For this review, take the finished solid that the model builds, in its own axes (mm). A direction names the side the tool comes from. Give positions to 0.01 mm unless a question says otherwise; leave off trailing zeros. Write each loop counter-clockwise with the first axis right and the second up, starting at its lowest first coordinate (ties: lowest second). Pieces come first, ordered by that corner, then holes.
Q1. For line 1 (Z direction, x = 10, y = -5.75); line 2 (Y direction, x = 14.5, z = 4.25); line 3 (X direction, y = 1, z = 14.5), list the stretches that pass through material, from the lowest coordinate up.
Q2. We need section B-B (x = 10). Write out the cut boundary in (y, z).
Q3. We need section C-C (x = -7.5). Write out the cut boundary in (y, z), then the cut area to 3 significant figures.
Q4. Mouldability with a two-part tool opening along Z and no side actions: class faces 3 (the cylindrical face through (12.75, 8.4, 9.86)), 4 (the flat face through (0, 0, 0)), 5 (the cylindrical face through (-2.899, -13.521, 10.083)), 6 (the cylindrical face through (-15.045, -13.521, 3.873)) as released by +Z, released by -Z, zero draft, split by the parting line, or undercut.
Q5. We need section A-A (z = 10.5). Give the number of separate pieces and of enclosed holes in the cut face, then the cut area to 3 significant figures.
Q6. Machinability: for faces 1 (the cylindrical face through (12.85, -8.04, 9.86)), 2 (the flat face through (0, 2, 11)), which of the approach directions +Z, -Z, +X, -X, +Y, -Y give a long, thin tool a straight path to every point of the face, cutting with its end or side? Answer none if there is none.
Q7. Insertion check: P1, Ø5.5, axis at x = -14.4, z = 6.8, coming from the +Y side; P2, Ø16, axis at x = -14.5, y = 3.5, coming from the +Z side; P3, Ø1, axis at y = -10, z = 11, coming from the -X side. Each pin has a flat end and moves straight along its axis. Give the tip position at first contact, or say it passes through.
Q8. We need section D-D (x = 6). Write out the cut boundary in (y, z).
```python
from build123d import *

# Parameters (mm, degrees)
F0_W     = 20
F0_H     = 27
F0_R     = 3
F0_R_2   = 2.75
F0_R_3   = 2.5
F1_DEPTH = 3
F0_R_4   = 1.55
F0_R_5   = 1.6
F0_R_6   = 1.5
F0_R_7   = 1.65
F0_R_8   = 1.45
F0_R_9   = 1.7
F2_DEPTH = 20
F0_H_2   = 3
F3_DEPTH = 20
F4_R     = 1.4
F4_R_2   = 1.45
F4_R_3   = 1.5
F4_R_4   = 2.75
F4_R_5   = 2.5
F4_R_6   = 3
F5_DEPTH = 30


with BuildPart() as f1:
    # F0 (on Top) → F1 (new body)
    with BuildSketch(Plane.XY):
        with Locations((-10, 1.5)):
            Rectangle(F0_W, F0_H)
        with Locations((-13.873821, -1.985078)):
            Circle(F0_R, mode=Mode.SUBTRACT)
        with Locations((-5.548216, 2.859571)):
            Circle(F0_R_2, mode=Mode.SUBTRACT)
        with Locations((-13.873821, 8.230659)):
            Circle(F0_R_3, mode=Mode.SUBTRACT)
    extrude(amount=F1_DEPTH)

    # F0 (on Top) → F2 (join)
    with BuildSketch(Plane.XY):
        Polygon((0, -15), (20, -15), (20, 15), (0, 15), (0, -12), align=None)
        with Locations((6.521292, -8.111834)):
            Circle(F0_R_4, mode=Mode.SUBTRACT)
        with Locations((14.447207, -8.111834)):
            Circle(F0_R_5, mode=Mode.SUBTRACT)
        with Locations((6.521292, 0)):
            Circle(F0_R_6, mode=Mode.SUBTRACT)
        with Locations((14.447207, 0)):
            Circle(F0_R_7, mode=Mode.SUBTRACT)
        with Locations((6.521292, 8.330117)):
            Circle(F0_R_8, mode=Mode.SUBTRACT)
        with Locations((14.447207, 8.330117)):
            Circle(F0_R_9, mode=Mode.SUBTRACT)
    extrude(amount=F2_DEPTH)

    # F0 (on Top) → F3 (join, through all)
    with BuildSketch(Plane.XY):
        with Locations((-10, -13.5)):
            Rectangle(F0_W, F0_H_2)
    extrude(amount=F3_DEPTH)

    # F4 (on face) → F5 (cut, through all)
    with BuildSketch(Plane.XZ.offset(15)):
        with Locations((10, 15.604385)):
            Circle(F4_R)
        with Locations((10, 10)):
            Circle(F4_R_2)
        with Locations((10, 4.171362)):
            Circle(F4_R_3)
        with Locations((-5.521618, 9.25734)):
            Circle(F4_R_4)
        with Locations((-11.956942, 14.9168)):
            Circle(F4_R_5)
        with Locations((-14.395144, 6.801534)):
            Circle(F4_R_6)
    extrude(amount=-F5_DEPTH, mode=Mode.SUBTRACT)


solid = f1.part
```
Computed:
1. line 1: z = 0 to 2.67, 5.67 to 8.55, 11.45 to 14.2, 17 to 20
1. line 2: y = -15 to -9.71, -6.51 to -1.65, 1.65 to 6.63, 10.03 to 15
1. line 3: x = 0 to 5.4, 7.64 to 9.14, 10.86 to 13.13, 15.76 to 20
2. outline: (-15, 0) - (15, 0) - (15, 2.67) - (-15, 2.67) - close; (-15, 5.67) - (15, 5.67) - (15, 8.55) - (-15, 8.55) - close; (-15, 11.45) - (15, 11.45) - (15, 14.2) - (-15, 14.2) - close; (-15, 17) - (15, 17) - (15, 20) - (-15, 20) - close
3. outline: (-15, 0) - (0.92, 0) - (0.92, 3) - (-12, 3) - (-12, 7.35) - (-15, 7.35) - close; (-15, 11.17) - (-12, 11.17) - (-12, 20) - (-15, 20) - close; (4.8, 0) - (15, 0) - (15, 3) - (4.8, 3) - close
3. area: 118 mm2
4. face 3: zero draft
4. face 4: released by -Z
4. face 5: undercut
4. face 6: undercut
5. separate pieces: 3
5. enclosed holes: 6
5. area: 517 mm2
6. face 1: +Z, -Z
6. face 2: +Z, -X, +Y
7. P1: passes through
7. P2: stops at z = 3
7. P3: stops at x = 0
8. outline: (-15, 0) - (-9.57, 0) - (-9.57, 20) - (-15, 20) - close; (-6.65, 0) - (-1.41, 0) - (-1.41, 20) - (-6.65, 20) - close; (1.41, 0) - (6.98, 0) - (6.98, 20) - (1.41, 20) - close; (9.68, 0) - (15, 0) - (15, 20) - (9.68, 20) - close
